Answer from the drawing. Dimensions are ordinates in mm from the lowest x, y and z of the part. Round coordinates to 2 decimals unless told otherwise and drop trailing zeros. Loops run counter-clockwise (first coordinate to the right, second up) from the corner with the lowest first, then second, coordinate; pieces in that order, holes last. Notation, with made-up numbers: (68.25, -26) - (73.25, -26) arc R32 ccw to (73.25, 5) - close; hole circle Ø5 at (-2, 13). An arc over 180 degrees is marked (long way). Return JSON: item names as keys, results as strings.
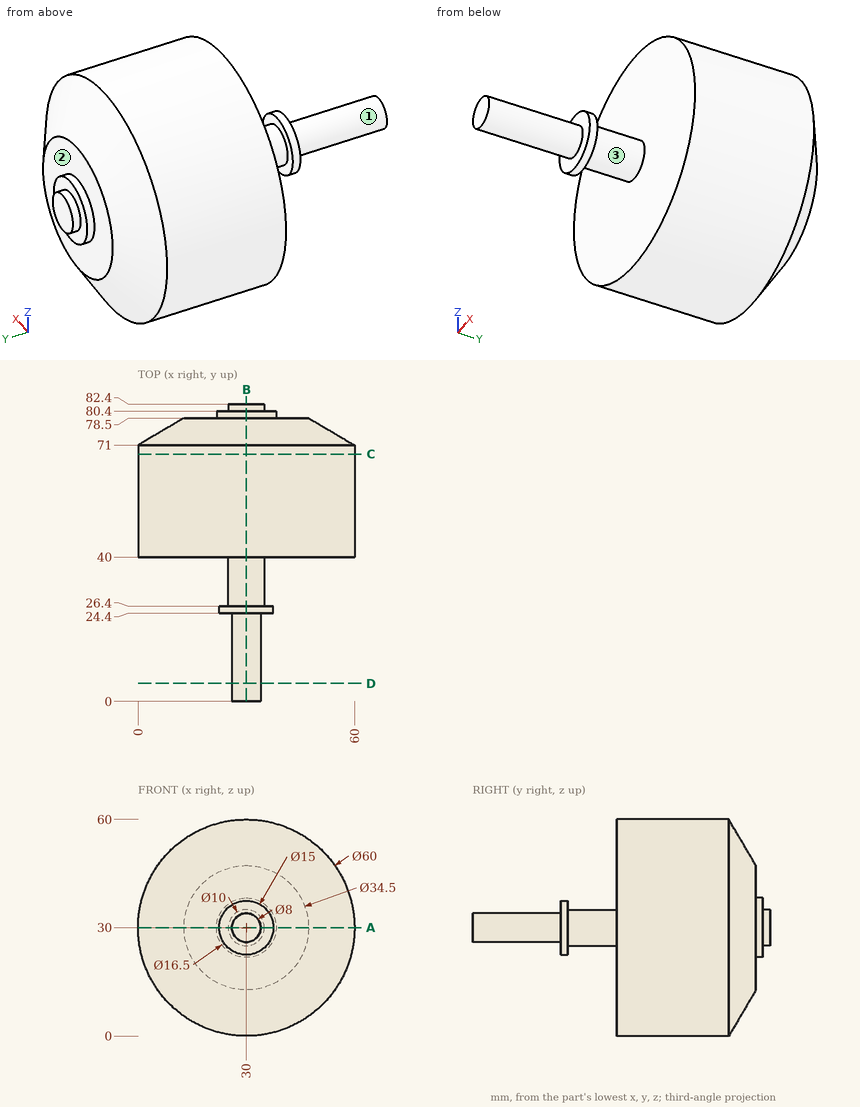
1) Section C-C (y = 68.5) is taken. Give the vertices of the cut face in (x, z), and give its area (3 significant figures).
Verdict:
{"outline": "circle Ø60 at (30, 30)", "area": "2,830 mm2"}
2) Find the intervals of material crossed by L1, parallel to Y at x = 24.5, z = 30; L2, parallel to Y at x = 22.5, z = 35.5; L3, parallel to Z at x = 31, y = 58, in increasing order.
Verdict:
{"L1": "y = 24.4 to 26.4, 40 to 80.4", "L2": "y = 40 to 78.5", "L3": "z = 0.02 to 59.98"}
3) Section A-A (z = 30) is taken. Give the vertices of the cut face in (x, y), and give its area (3 significant figures).
Verdict:
{"outline": "(0, 40) - (25, 40) - (25, 26.4) - (22.5, 26.4) - (22.5, 24.4) - (26, 24.4) - (26, 0) - (34, 0) - (34, 24.4) - (37.5, 24.4) - (37.5, 26.4) - (35, 26.4) - (35, 40) - (60, 40) - (60, 71) - (47.25, 78.5) - (38.25, 78.5) - (38.25, 80.4) - (35, 80.4) - (35, 82.4) - (25, 82.4) - (25, 80.4) - (21.75, 80.4) - (21.75, 78.5) - (12.75, 78.5) - (0, 71) - close", "area": "2,630 mm2"}
4) Section D-D (y = 5) is taken. Give the vertices of the cut face in (x, z), and give its area (3 significant figures).
Verdict:
{"outline": "circle Ø8 at (30, 30)", "area": "50.3 mm2"}
5) Flat-ended cylindrical pins translate along their axes: pin 1 (2 mm diameter, centred on x = 8.5, z = 44, fed in from -Y); pin 2 (16.5 mm diameter, centred on x = 30, z = 27.5, fed in from -Y); pin 3 (12 mm diameter, centred on y = 62, z = 44, fed in from +X); pin 4 (5 mm diameter, centred on y = 65.5, z = 40.5, fed in from -X). Find the tip coordinate at first contact, or state that the pin passes through.
Verdict:
{"pin 1": "stops at y = 40", "pin 2": "stops at y = 0", "pin 3": "stops at x = 58.91", "pin 4": "stops at x = 1.09"}
6) Section B-B (x = 30) is taken. Give the vertices of the cut face in (y, z), and give its area (3 significant figures).
Verdict:
{"outline": "(0, 26) - (24.4, 26) - (24.4, 22.5) - (26.4, 22.5) - (26.4, 25) - (40, 25) - (40, 0) - (71, 0) - (78.5, 12.75) - (78.5, 21.75) - (80.4, 21.75) - (80.4, 25) - (82.4, 25) - (82.4, 35) - (80.4, 35) - (80.4, 38.25) - (78.5, 38.25) - (78.5, 47.25) - (71, 60) - (40, 60) - (40, 35) - (26.4, 35) - (26.4, 37.5) - (24.4, 37.5) - (24.4, 34) - (0, 34) - close", "area": "2,630 mm2"}
7) Determine the mould class of the marked faces 1, 2 and 3 for opening direction Y: pulls with the +Y half, pulls with the -Y half, needs draft (parallel to the pull), parting line crosses it, or undercut.
Verdict:
{"face 1": "needs draft", "face 2": "pulls with the +Y half", "face 3": "undercut"}
